For this review, use the dimensioned drawing (mm, ordinates from the lowest corner) and the shaded views. A direction names the side the tool comes from. Coordinates: 2 decimals unless noted, no trailing zeros. Loops run counter-clockwise (first coordinate to the right, second up) from the corner with the lowest first, then second, coordinate; pieces in that order, holes last. Notation, with made-up numbers: M 3,-8 L 44,-8 A28 cw 44,12 Z; hole C 14,43 d8. An arc over 180 degrees is marked long. One line per item, written item: value.
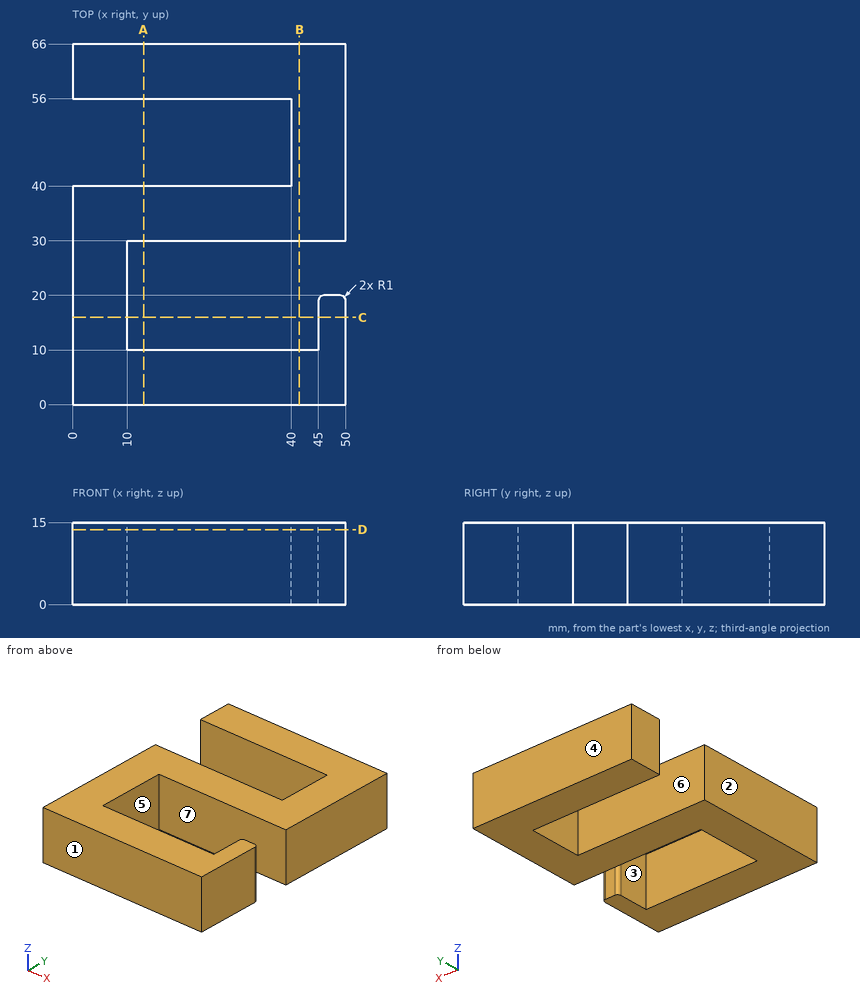
(1) Add section D-D on z = 13.75. State the section outline as (x, y) points, then the cut area to 3 significant figures.
Checks:
outline: M 0,0 L 50,0 L 50,19 A1 ccw 49,20 L 46,20 A1 ccw 45,19 L 45,10 L 10,10 L 10,30 L 50,30 L 50,66 L 0,66 L 0,56 L 40,56 L 40,40 L 0,40 Z
area: 1,910 mm^2
(2) Draft analysis for pull direction Y (two halves, no side actions). For the marked faces 1, 2, 3 and 4, state which applies: pulls with the +Y half, pulls with the -Y half, needs draft (parallel to the pull), parting line crosses it, or undercut.
Checks:
face 1: pulls with the -Y half
face 2: needs draft
face 3: undercut
face 4: pulls with the +Y half
(3) To check wall thickness, follow L1, parallel to Y at x = 24, z = 8.75; L2, parallel to Y at x = 43.5, z = 13.25; L3, parallel to X at y = 14, z = 5.25. State the ranges of each line that lie inside material, in increasing order. Write a range as [from, to].
Checks:
L1: [0, 10], [30, 40], [56, 66]
L2: [0, 10], [30, 66]
L3: [0, 10], [45, 50]
(4) Insertion check: pin 1 Ø1 at (x, z) = (21.5, 3.5) entering from -Y; pin 2 Ø2 at (x, y) = (42, 11.5) entering from +Z; pin 3 Ø4.5 at (y, z) = (44, 4.5) entering from -X. Each pin has a flat end and moves straight along its axis. Give the tip position at first contact, or say it passes through.
Checks:
pin 1: y = 0
pin 2: through
pin 3: x = 40
(5) Add section B-B on x = 41.5. State the section outline as (y, z) points, then the cut area to 3 significant figures.
Checks:
outline: M 0,0 L 10,0 L 10,15 L 0,15 Z; M 30,0 L 66,0 L 66,15 L 30,15 Z
area: 690 mm^2
(6) Add section A-A on x = 13. State the section outline as (y, z) points, then the cut area to 3 significant figures.
Checks:
outline: M 0,0 L 10,0 L 10,15 L 0,15 Z; M 30,0 L 40,0 L 40,15 L 30,15 Z; M 56,0 L 66,0 L 66,15 L 56,15 Z
area: 450 mm^2
(7) Tool access review of the marked faces 5, 6 and 7: name each direction out of +Z, -Z, +X, -X, +Y, -Y from which nothing blocks a thin tool from reaching the whole face with its end or side.
Checks:
face 5: +Z, -Z
face 6: +Z, -Z, -X
face 7: +Z, -Z, +X
(8) Add section C-C on y = 16. State the section outline as (x, z) points.
Checks:
outline: M 0,0 L 10,0 L 10,15 L 0,15 Z; M 45,0 L 50,0 L 50,15 L 45,15 Z
